Geometry check sheet. Reference: the model listing, model coordinates, mm. A direction names the side the tool comes from. Round coordinates to 2 decimals unless told otherwise and drop trailing zeros. Write each loop counter-clockwise with the first axis right and the second up, starting at its lowest first coordinate (ties: lowest second). Pieces come first, ordered by that corner, then holes. Notation, with made-up numbers: M 16.25,48 L 56.25,48 A7 cw 56.25,57 Z; hole C 62.5,50 d9. An arc over 180 degrees is marked long. Use a Markdown table: item, result.
```python
from build123d import *

# Parameters (mm, degrees)
ESQUISSE1_R             = 20
ESQUISSE1_R_2           = 15
BOSS_EXTRU_1_DEPTH      = 22
ESQUISSE5_R             = 15
BOSS_EXTRU_3_DEPTH      = 2.5
ESQUISSE12_R            = 4.25
ENL_V_MAT_EXTRU_2_DEPTH = 2.5


with BuildPart() as part:
    # Esquisse1 → Boss.-Extru.1 (new body)
    with BuildSketch(Plane.XY):
        Circle(ESQUISSE1_R)
        Circle(ESQUISSE1_R_2, mode=Mode.SUBTRACT)
    extrude(amount=BOSS_EXTRU_1_DEPTH)

    # Esquisse5 → Boss.-Extru.3 (add)
    with BuildSketch(Plane(origin=(0, 0, 0), x_dir=(-1, 0, 0), z_dir=(0, 0, -1))):
        Circle(ESQUISSE5_R)
    extrude(amount=-BOSS_EXTRU_3_DEPTH)

    # Esquisse12 → Enlèv. mat.-Extru.2 (cut)
    with BuildSketch(Plane(origin=(0, 0, 0), x_dir=(-1, 0, 0), z_dir=(0, 0, -1))):
        Circle(ESQUISSE12_R)
    extrude(amount=-ENL_V_MAT_EXTRU_2_DEPTH, mode=Mode.SUBTRACT)


solid = part.part
```
Item 1: Mould release check, pull along X, two halves, no side actions. Record for faces 3 (the face through (0, 5, 0)), 4 (the face through (-2.285, 3.584, 1.232)), 5 (the face through (-4.336, -19.524, 10.846)): +X half, -X half, draft (parallel to the pull), parting line (faces both ways), or undercut.
Outcome:
| item | result |
|---|---|
| face 3 | draft |
| face 4 | undercut |
| face 5 | parting line |
Item 2: Go/stop test with flat-tipped pins: pin 1 (2 mm diameter, centred on x = 2, y = 4.5, fed in from -Z); pin 2 (4 mm diameter, centred on y = -11.5, z = 16.5, fed in from +X); pin 3 (13.5 mm diameter, centred on x = 0, y = 0, fed in from +Z); pin 4 (1 mm diameter, centred on x = -3.5, z = 15, fed in from +Y). Record where each tip stops, or that it passes through.
Outcome:
| item | result |
|---|---|
| pin 1 | stops at z = 0 |
| pin 2 | stops at x = 17.6 |
| pin 3 | stops at z = 2.5 |
| pin 4 | stops at y = 19.77 |
Item 3: Cross-section at D-D, the plane y = -5. Record the cut outline in (x, z).
Outcome:
| item | result |
|---|---|
| outline | M -19.36,0 L 19.36,0 L 19.36,22 L 14.14,22 L 14.14,2.5 L -14.14,2.5 L -14.14,22 L -19.36,22 Z |
Item 4: Access from +Z, -Z, +X, -X, +Y, -Y to the whole of each face (thin tool, end or side, straight path). Record for faces 1 (the face through (-14.985, 0.66, 12.114)), 2 (the face through (3, 15, 22)).
Outcome:
| item | result |
|---|---|
| face 1 | +Z |
| face 2 | +Z, +X, -X, +Y, -Y |
Item 5: Cross-section at C-C, the plane z = 20.5. Record the cut outline in (x, y).
Outcome:
| item | result |
|---|---|
| outline | C 0,0 d40; hole C 0,0 d30 |
Item 6: Cross-section at A-A, the plane y = 0. Record the cut outline in (x, z), and give its area (3 significant figures).
Outcome:
| item | result |
|---|---|
| outline | M -20,0 L -4.25,0 L -4.25,2.5 L -15,2.5 L -15,22 L -20,22 Z; M 4.25,0 L 20,0 L 20,22 L 15,22 L 15,2.5 L 4.25,2.5 Z |
| area | 274 mm2 |
Item 7: Material ranges on line 1 along Y through (x, z) = (0, 1.05); line 2 along Y through (x, z) = (0, 6.5); line 3 along X through (y, z) = (0.5, 7), recorded low to high. Write a range as from..to.
Outcome:
| item | result |
|---|---|
| line 1 | y = -20..-4.25, 4.25..20 |
| line 2 | y = -20..-15, 15..20 |
| line 3 | x = -19.99..-14.99, 14.99..19.99 |
